Geometry check sheet. Reference: the model listing, model coordinates, mm. Face numbers are marked on the shaded views. A direction names the side the tool comes from. Coordinates: 2 decimals unless noted, no trailing zeros. Order: outer loops, then holes, each group sorted by start corner. A loop starts at its lowest first (then second) coordinate and runs counter-clockwise, first axis right, second up. Notation, with made-up numbers: (-1, 29.25) -> (45, 29.25) arc R22 ccw to (45, 63.25) -> close; hole circle Ø7 at (-4, -32). An arc over 180 degrees is marked (long way). Answer in a Markdown table with one row per item. Add a question column.
Solid Edge part; units mm, degrees
sketch "Sketch1" plane through (0, 0, 0) normal (0, 0, 1) x (1, 0, 0)
  circle A0 centre (0, 0) radius 40
extrude "Protrusion1" add sketch "Sketch1" along normal blind 14
sketch "Sketch2" plane through (0, 0, 0) normal (0, 0, 1) x (1, 0, 0)
  line L0 (-37.081, 15) -> (-37.081, -15)
extrude "Cutout1" cut sketch "Sketch2" along normal through all material side at (-37.131, 0, 0)
sketch "Sketch3" plane through (-37.081, 0, 6) normal (-1, 0, 0) x (0, -1, 0)
  line L0 (14.4, 5) -> (-14.4, 5)
  line L1 (-14.4, 5) -> (-14.4, -3)
  line L2 (-14.4, -3) -> (14.4, -3)
  line L3 (14.4, -3) -> (14.4, 5)
extrude "Extrusionsausschnitt_5" cut sketch "Sketch3" against normal blind 22
sketch "Sketch4" plane through (-24.581, 0, 3) normal (0, 0, 1) x (0, -1, 0)
  line L0 (-7.5, 7.5) -> (-7.5, -7.5)
  line L1 (-7.5, -7.5) -> (-11, -7.5)
  line L2 (-11, -7.5) -> (-11, 7.5)
  line L3 (-11, 7.5) -> (-7.5, 7.5)
extrude "Cutout2" cut sketch "Sketch4" against normal through all
mirror "Mirror1" about plane through (0, 0, 0) normal (0, -1, 0) of "Cutout2"
pattern_circular "Pattern1" count 3 over 360 about axis through (0, 0, 0) along (0, 0, -1) of "Mirror1", "Cutout2", "Extrusionsausschnitt_5", "Cutout1"
hole "Bohrung_3" at (12, 0, 0) direction (0, 0, 1) diameter 3.2 end through all
hole "Hole1" at (24, 0, 0) direction (0, 0, 1) diameter 3.2 end through all
hole "Bohrung_5" at (-12, 0, 0) direction (0, 0, 1) diameter 3.2 end through all
hole "Bohrung_6" at (-11, 32, 0) direction (0, 0, 1) diameter 2.7 end through all
hole "Hole2" at (-11, -32, 0) direction (0, 0, 1) diameter 2.7 end through all
hole "Bohrung_8" at (-12, 0, 0) direction (0, 0, 1) diameter 7 depth 1
hole "Hole3" at (12, 0, 0) direction (0, 0, 1) diameter 7 depth 1
hole "Hole4" at (24, 0, 0) direction (0, 0, 1) diameter 7 depth 1
properties material "PLA(50%)"
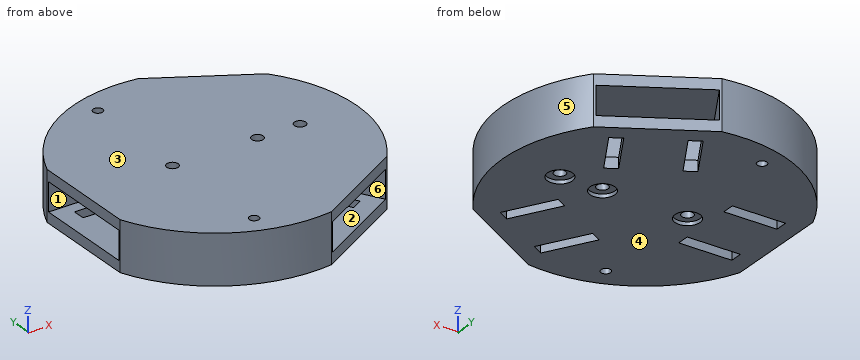
(1) Access from +Z, -Z, +X, -X, +Y, -Y to the whole of each face (thin tool, end or side, straight path). Record for the marked faces 1, 2 and 3.
(2) Cross-section at D-D (x = 12). Enter the section's corners in (y, z), plus the area to 3 significant figures.
(3) Cross-section at A-A (y = 0). Give the number of separate pieces and of enclosed holes in the cut face, plus the area to 3 significant figures.
(4) Scan lines: line 1 along X through (y, z) = (0, 0.3); line 2 along X through (y, z) = (0, 10.75); line 3 along Y through (x, z) = (-11, 8.5). Record each from-to range of solid material in increasing order.
(5) Cross-section at C-C (x = 24). Enter the section's corners in (y, z), plus the area to 3 significant figures.
(6) Go/stop test with flat-tipped pins: P1, Ø1.5, axis at x = -19, z = 5.5, coming from the +Y side; P2, Ø16.5, axis at x = 14.5, y = -16, coming from the -Z side; P3, Ø6.5, axis at x = -25, z = 7, coming from the -Y side; P4, Ø4, axis at x = -30.5, z = 6.5, coming from the +Y side. Record where each tip stops, or that it passes through.
(7) Cross-section at B-B (z = 7.25). Enter the section's corners in (x, y).
(8) Mould release check, pull along X, two halves, no side actions. Record for the marked faces 4, 5 and 6: +X half, -X half, draft (parallel to the pull), parting line (faces both ways), or undercut.
Checks:
| question | item | result |
|---|---|---|
| 1 | face 1 | -X |
| 1 | face 2 | none |
| 1 | face 3 | +Z, +X, -X, +Y, -Y |
| 2 | outline | (-35.89, 0) -> (-3.5, 0) -> (-3.5, 1) -> (-1.6, 1) -> (-1.6, 14) -> (-35.89, 14) -> (-35.89, 11) -> (-10.49, 11) -> (-10.49, 3) -> (-35.89, 3) -> close; (1.6, 1) -> (3.5, 1) -> (3.5, 0) -> (35.89, 0) -> (35.89, 3) -> (10.49, 3) -> (10.49, 11) -> (35.89, 11) -> (35.89, 14) -> (1.6, 14) -> close |
| 2 | area | 550 mm² |
| 3 | separate pieces | 4 |
| 3 | enclosed holes | 0 |
| 3 | area | 757 mm² |
| 4 | line 1 | -37.08 to -15.5, -8.5 to 8.5, 15.5 to 20.5, 27.5 to 40 |
| 4 | line 2 | -15.08 to -13.6, -10.4 to 10.4, 13.6 to 22.4, 25.6 to 40 |
| 4 | line 3 | -38.46 to -33.35, -30.65 to -1.25, 1.25 to 30.65, 33.35 to 38.46 |
| 5 | outline | (-28.96, 0) -> (-23.19, 0) -> (-23.19, 3) -> (-28.96, 3) -> close; (-28.96, 11) -> (-12.77, 11) -> (-12.77, 3) -> (-19.57, 3) -> (-19.57, 0) -> (-3.5, 0) -> (-3.5, 1) -> (-1.6, 1) -> (-1.6, 14) -> (-28.96, 14) -> close; (1.6, 1) -> (3.5, 1) -> (3.5, 0) -> (19.57, 0) -> (19.57, 3) -> (12.77, 3) -> (12.77, 11) -> (28.96, 11) -> (28.96, 14) -> (1.6, 14) -> close; (23.19, 0) -> (28.96, 0) -> (28.96, 3) -> (23.19, 3) -> close |
| 5 | area | 482 mm² |
| 6 | P1 | y = 35.59 |
| 6 | P2 | z = 0 |
| 6 | P3 | y = -33.57 |
| 6 | P4 | y = 28.07 |
| 7 | outline | (-37.08, -15) arc R40 ccw to (5.55, -39.61) -> (6.07, -39.31) -> (-4.93, -20.26) -> (20.01, -5.86) -> (31.01, -24.91) -> (31.53, -24.61) arc R40 ccw to (31.53, 24.61) -> (31.01, 24.91) -> (20.01, 5.86) -> (-4.93, 20.26) -> (6.07, 39.31) -> (5.55, 39.61) arc R40 ccw to (-37.08, 15) -> (-37.08, 14.4) -> (-15.08, 14.4) -> (-15.08, -14.4) -> (-37.08, -14.4) -> close; hole circle Ø3.2 at (-12, 0); hole circle Ø2.7 at (-11, -32); hole circle Ø2.7 at (-11, 32); hole circle Ø3.2 at (12, 0); hole circle Ø3.2 at (24, 0) |
| 8 | face 4 | draft |
| 8 | face 5 | +X half |
| 8 | face 6 | undercut |
